Study the drawing (mm; zero at the part's minimum x, y, z) and answer. A direction names the side the tool comes from. Give positions to 0.01 mm unless a question says otherwise; leave off trailing zeros.
1) Straight lines are drawn through the part: probe 1 along Y at (x, z) = (48.5, 29.5); probe 2 along Y at (x, z) = (61, 16.5); probe 3 along Y at (x, z) = (4.75, 12.7). For each, find the intervals that lie inside material, in ascending order.
2) Find section D-D (z = 7.5). Count the separate pieces of the cut face and the enclosed holes in it, plus the area to 3 significant figures.
3) Determine the mould class of the marked faces 1, 2 and 3 for opening direction Z: pulls with the +Z half, pulls with the -Z half, needs draft (parallel to the pull), parting line crosses it, or undercut.
4) A tool of negligible diameter and unlimited length cuts with its end or side. For the marked faces 4 and 5, from which of +Z, -Z, +X, -X, +Y, -Y can it reach the whole face along a straight path? Write none if from no direction.
5) Given pin 1 Ø3 at (y, z) = (3.5, 48.5) entering from -X; pin 2 Ø8 at (x, z) = (39, 21) entering from +Y; pin 3 Ø4 at (x, z) = (60, 34) entering from +Y, each flat-ended and moving along its own axis, determine where each tip first touches the part or whether it passes through.
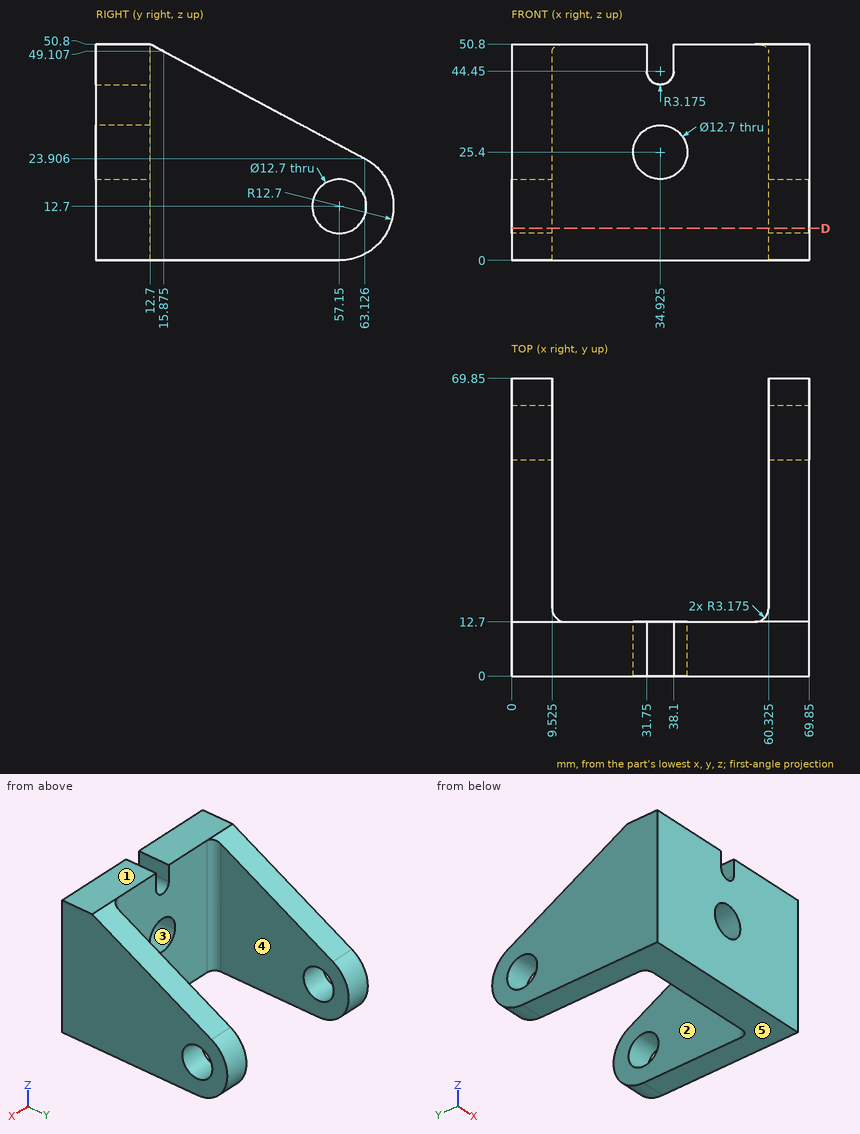
Results:
1. probe 1: y = 0 to 12.7
1. probe 2: y = 0 to 52.06, 62.24 to 69.27
1. probe 3: y = 0 to 50.8, 63.5 to 69.85
2. separate pieces: 3
2. enclosed holes: 0
2. area: 1,820 mm2
3. face 1: pulls with the +Z half
3. face 2: needs draft
3. face 3: undercut
4. face 4: +Z, -Z, +Y
4. face 5: -Z, +X, -X, +Y, -Y
5. pin 1: stops at x = 0
5. pin 2: stops at y = 12.7
5. pin 3: stops at y = 47.9
